```python
from build123d import *

# Parameters (mm, degrees)
SKETCH_1_W          = 39
SKETCH_1_H          = 20
SKETCH_1_R          = 1.6
EXTRUDE_1_DEPTH     = 3
SKETCH_2_W          = 39
SKETCH_2_H          = 3
EXTRUDE_2_DEPTH     = 4
SKETCH_3_R          = 1.6
CUT_EXTRUDE_1_DEPTH = 4


with BuildPart() as part:
    # ｽｹｯﾁ1 → ﾎﾞｽ - 押し出し1 (new body)
    with BuildSketch(Plane.XY):
        Rectangle(SKETCH_1_W, SKETCH_1_H)
        with Locations((15.5, 6)):
            Circle(SKETCH_1_R, mode=Mode.SUBTRACT)
        with BuildLine():
            ThreePointArc((-15.5, 7.6), (-14.36862915, 4.86862915), (-17.1, 6))
            Line((-17.1, 6), (-15.5, 6))
            Line((-15.5, 6), (-15.5, 7.6))
        make_face(mode=Mode.SUBTRACT)
    extrude(amount=EXTRUDE_1_DEPTH)

    # ｽｹｯﾁ2 → ﾎﾞｽ - 押し出し2 (add)
    with BuildSketch(Plane.XZ.offset(10)):
        with Locations((0, 1.5)):
            Rectangle(SKETCH_2_W, SKETCH_2_H)
    extrude(amount=EXTRUDE_2_DEPTH)

    # ｽｹｯﾁ3 → ｶｯﾄ - 押し出し1 (cut)
    with BuildSketch(Plane.XY.offset(3)):
        with Locations((-15.5, 6)):
            Circle(SKETCH_3_R)
        with Locations((-15.5, -10)):
            Circle(SKETCH_3_R)
        with Locations((15.5, -10)):
            Circle(SKETCH_3_R)
    extrude(amount=-CUT_EXTRUDE_1_DEPTH, mode=Mode.SUBTRACT)


solid = part.part
```
For this review, take the finished solid that the model builds, in its own axes (mm). Give positions to 0.01 mm unless a question says otherwise; leave off trailing zeros. Write each loop counter-clockwise with the first axis right and the second up, starting at its lowest first coordinate (ties: lowest second). Pieces come first, ordered by that corner, then holes. Notation, with made-up numbers: M 25.25,-30.75 L 78.25,-30.75 A18 ccw 78.25,-20.75 Z; hole C 56.5,-25.75 d9. An arc over 180 degrees is marked long. Answer as a JSON object with one key per item and string values. Group by question number.
Item 1: Consider section C-C on x = 15.5. Write out the cut boundary in (y, z), plus the area to 3 significant figures.
Item 2: Draft analysis for pull direction Y (two halves, no side actions). For faces 1 (the cylindrical face through (13.9, 6.07, 1.48)), 2 (the flat face through (19.5, -2, 1)), 3 (the flat face through (0, -14, 2)), 4 (the cylindrical face through (14.23, -10.97, 1.52)), state which applies: +Y half, -Y half, draft (parallel to the pull), parting line (faces both ways), or undercut.
Item 3: For pin 1 Ø3 at (x, y) = (15.5, 6) entering from -Z, flat-tipped, find the tip position at first contact; note if it passes through.
Item 4: Consider section B-B on z = 2.4. Write out the cut boundary in (x, y).
Item 5: Consider section A-A on y = -10. Write out the cut boundary in (x, z).
Item 6: For probe 1 along Y at (x, z) = (-15.5, 1.65); probe 2 along X at (y, z) = (5, 2.15); probe 3 along X at (y, z) = (-10.25, 1.05), list the stretches that pass through material, from the lowest coordinate up. Write a range as [from, to].
Check result:
{
 "1": {"outline": "M -14,0 L -11.6,0 L -11.6,3 L -14,3 Z; M -8.4,0 L 4.4,0 L 4.4,3 L -8.4,3 Z; M 7.6,0 L 10,0 L 10,3 L 7.6,3 Z", "area": "52.8 mm^2"},
 "2": {"face 1": "undercut", "face 2": "draft", "face 3": "-Y half", "face 4": "undercut"},
 "3": {"pin 1": "passes through"},
 "4": {"outline": "M -19.5,-14 L 19.5,-14 L 19.5,10 L -19.5,10 Z; hole C -15.5,-10 d3.2; hole C -15.5,6 d3.2; hole C 15.5,-10 d3.2; hole C 15.5,6 d3.2"},
 "5": {"outline": "M -19.5,0 L -17.1,0 L -17.1,3 L -19.5,3 Z; M -13.9,0 L 13.9,0 L 13.9,3 L -13.9,3 Z; M 17.1,0 L 19.5,0 L 19.5,3 L 17.1,3 Z"},
 "6": {"probe 1": "y = [-14, -11.6], [-8.4, 4.4], [7.6, 10]", "probe 2": "x = [-19.5, -16.75], [-14.25, 14.25], [16.75, 19.5]", "probe 3": "x = [-19.5, -17.08], [-13.92, 13.92], [17.08, 19.5]"}
}
